from build123d import *

# Parameters (mm, degrees)
SKETCH2_W           = 600
SKETCH2_H           = 350
BOSS_EXTRUDE1_DEPTH = 3
SKETCH3_W           = 450
SKETCH3_H           = 350
BOSS_EXTRUDE2_DEPTH = 125
SKETCH4_R           = 10
CUT_EXTRUDE1_DEPTH  = 350
SKETCH6_R           = 5
CUT_EXTRUDE2_DEPTH  = 20
SKETCH7_W           = 120
SKETCH7_H           = 120.57779395
SKETCH7_R           = 3
BOSS_EXTRUDE3_DEPTH = 1


with BuildPart() as part:
    # Sketch2 → Boss-Extrude1 (new body)
    with BuildSketch(Plane(origin=(0, 0, 0), x_dir=(1, 0, 0), z_dir=(0, 1, 0))):
        Rectangle(SKETCH2_W, SKETCH2_H)
    extrude(amount=BOSS_EXTRUDE1_DEPTH)

    # Sketch3 → Boss-Extrude2 (add)
    with BuildSketch(Plane(origin=(0, 3, 0), x_dir=(1, 0, 0), z_dir=(0, 1, 0))):
        with Locations((75, 0)):
            Rectangle(SKETCH3_W, SKETCH3_H)
    extrude(amount=BOSS_EXTRUDE2_DEPTH)

    # Sketch4 → Cut-Extrude1 (cut)
    with BuildSketch(Plane.XY.offset(175)):
        with Locations((0, 44)):
            Circle(SKETCH4_R)
    extrude(amount=-CUT_EXTRUDE1_DEPTH, mode=Mode.SUBTRACT)

    # Sketch6 → Cut-Extrude2 (cut)
    with BuildSketch(Plane(origin=(0, 128, 0), x_dir=(1, 0, 0), z_dir=(0, 1, 0))):
        with Locations(Location((150, 0, 0), (0, 0, 270))):
            Circle(SKETCH6_R)
    extrude(amount=-CUT_EXTRUDE2_DEPTH, mode=Mode.SUBTRACT)

    # Sketch7 → Boss-Extrude3 (add, symmetric)
    with BuildSketch(Plane(origin=(0, 3, 0), x_dir=(1, 0, 0), z_dir=(0, 1, 0))):
        with Locations((-240, 0.288896975)):
            Rectangle(SKETCH7_W, SKETCH7_H)
        with Locations(Location((-190, 50.57779395, 0), (0, 0, 270))):
            Circle(SKETCH7_R, mode=Mode.SUBTRACT)
        with Locations(Location((-290, -50, 0), (0, 0, 270))):
            Circle(SKETCH7_R, mode=Mode.SUBTRACT)
    extrude(amount=BOSS_EXTRUDE3_DEPTH, both=True)


solid = part.part
Model file for the job. Use its own axes, mm. A direction names the side the tool comes from. Round coordinates to 2 decimals unless told otherwise and drop trailing zeros. Loops run counter-clockwise (first coordinate to the right, second up) from the corner with the lowest first, then second, coordinate; pieces in that order, holes last.
1. Mould opens along Y. For faces 3 (the cylindrical face through (-2.17, 34.24, 2.45)), 4 (the flat face through (-4, 0, -2)), 5 (the flat face through (72, 128, -2)), 6 (the flat face through (-150, 65, 2)) say: +Y half, -Y half, draft (parallel to the pull), parting line (faces both ways), or undercut.
Check values:
face 3: undercut
face 4: -Y half
face 5: +Y half
face 6: draft
2. Band-saw the part on A-A, the plane x = 0. List the corners of the cut face in (y, z).
Check values:
outline: (0, -175) - (34, -175) - (34, 175) - (0, 175) - close; (54, -175) - (128, -175) - (128, 175) - (54, 175) - close
3. Wall check: probe 1 along Y at (x, z) = (0, -127); probe 2 along X at (y, z) = (3.65, 50); probe 3 along X at (y, z) = (118, 0). Give the ranges that are in metal, low to high.
Check values:
probe 1: y = 0 to 34, 54 to 128
probe 2: x = -300 to -293, -287 to -180, -150 to 300
probe 3: x = -150 to 145, 155 to 300
4. Band-saw the part on C-C, the plane y = 115. List the corners of the cut face in (x, z), and give its area (3 significant figures).
Check values:
outline: (-150, -175) - (300, -175) - (300, 175) - (-150, 175) - close; hole circle Ø10 at (150, 0)
area: 157,000 mm2
5. Tool access for faces 1 (the flat face through (-241, 4, -1)), 2 (the flat face through (300, 63, 2)): list every direction of +Z, -Z, +X, -X, +Y, -Y with a clear straight run to the whole face (end or side of a thin tool).
Check values:
face 1: +Z, -Z, -X, +Y
face 2: +Z, -Z, +X, +Y, -Y
6. Drop flat-ended pins along their axis: P1, Ø1.1, axis at x = -249, y = 3.5, coming from the -Z side; P2, Ø9.5, axis at x = -290, z = 50, coming from the +Y side; P3, Ø1.5, axis at y = 37, z = -126.5, coming from the -X side; P4, Ø5.5, axis at x = -190, z = -50.58, coming from the +Y side. Give the stop position or say it passes through.
Check values:
P1: stops at z = -175
P2: stops at y = 4
P3: stops at x = -150
P4: stops at y = 3
7. Band-saw the part on B-B, the plane z = -80.5. List the corners of the cut face in (x, y).
Check values:
outline: (-300, 0) - (300, 0) - (300, 128) - (-150, 128) - (-150, 3) - (-300, 3) - close; hole circle Ø20 at (0, 44)
